Autodesk Inventor part; units mm, degrees
ref_plane "YZ Plane" through (0, 0, 0) normal (1, 0, 0) x (0, 1, 0)
ref_plane "XZ Plane" through (0, 0, 0) normal (0, 1, 0) x (-1, 0, 0)
ref_plane "XY Plane" through (0, 0, 0) normal (0, 0, 1) x (1, 0, 0)
sketch "Sketch1" plane through (0, 0, 0) normal (0, 0, 1) x (1, 0, 0)
  line L0 (0, 1490) -> (-133.543, 1490)
  line L1 (-133.543, 1490) -> (-133.543, 0)
  line L2 (-133.543, 0) -> (0, 0)
  line L3 (0, 0) -> (0, 1490)
  line L4 (-133.543, 100) -> (-66, 100)
  line L5 (-66, 100) -> (-66, 105)
  line L6 (-66, 105) -> (-133.543, 105)
  line L7 (-133.543, 105) -> (-133.543, 100)
  line L8 (-133.543, 596.6667) -> (-66, 596.6667)
  line L9 (-66, 596.6667) -> (-66, 601.6667)
  line L10 (-66, 601.6667) -> (-133.543, 601.6667)
  line L11 (-133.543, 601.6667) -> (-133.543, 596.6667)
  line L12 (-133.543, 1093.3333) -> (-66, 1093.3333)
  line L13 (-66, 1093.3333) -> (-66, 1098.3333)
  line L14 (-66, 1098.3333) -> (-133.543, 1098.3333)
  line L15 (-133.543, 1098.3333) -> (-133.543, 1093.3333)
  circle A0 centre (-133.543, 1335) radius 30
  point P0 (-133.543, 105)
  point P1 (-133.543, 1365)
  point P2 (-133.543, 1305)
  dimension "d0" = 1490
  dimension "d1" = 133.543
  dimension "d2" = 5
  dimension "d4" = 100
  dimension "d7" = 496.6667
  dimension "d23" = 66
  dimension "d29" = 60
  dimension "d30" = 1335
extrude "Plate1" add sketch "Sketch1" along normal blind 4 contours L3 L2 L1 L4 L5 L6 L8 L9 L10 L12 L13 L14 A0 L0
chamfer "Corner Chamfer1" distance 3 angle 45 6 edges at (-133.543, 100, 2) (-133.543, 105, 2) (-133.543, 596.6667, 2) (-133.543, 601.6667, 2) (-133.543, 1098.3333, 2) (-133.543, 1093.3333, 2)
equation "\"d0\" = Стрингер_длина"
equation "\"d1\" = стрингер_глубина_6"
equation "\"d2\" = паз_под_стрингер_толщина"
equation "\"d7\" = Шаг_шпангоутов"
equation "\"d23\" = паз_под_стрингер_глубина - Thickness"
equation "\"d29\" = 2 * радиус_выреза_под_сварку"
equation "\"d12\" = Thickness"
equation "\"BendRadius\" = Thickness"
equation "\"BendReliefWidth\" = Thickness"
equation "\"BendReliefDepth\" = 0.5 * Thickness"
equation "\"CornerReliefSize\" = 4 * Thickness"
equation "\"MinimumRemnant\" = 2 * Thickness"
equation "\"TransitionRadius\" = BendRadius"
equation "\"JacobiRadiusSize\" = BendRadius"
equation "\"GapSize\" = Thickness"
properties part number "0715 GBK stringer C3" material "Steel"
Could you check a few things on this model? Use its own coordinates, in mm. Give positions to 0.01 mm unless a question says otherwise; leave off trailing zeros. Order: outer loops, then holes, each group sorted by start corner. A loop starts at its lowest first (then second) coordinate and runs counter-clockwise, first axis right, second up.
Q1. Suppose I cut it at A-A, the plane y = 1335. Write out the boundary of the cut face in (x, z).
Q2. If I drill on line 1 along Y through (x, z) = (-96.5, 3.6), over which ranges is the centre line in solid material (lowest first)?
Q3. I'm going to push a flat-ended pin straight in: P1, Ø2, axis at y = 1095.5, z = 2, coming from the -X side. Where does the tip first touch, or does it pass through?
Q4. We'd pull the mould along Y, two halves only. Please class faces 1 (the cylindrical face through (-103.55, 1335.66, 1.97)), 2 (the flat face through (-68, 755, 4)): +Y half, -Y half, draft (parallel to the pull), parting line (faces both ways), or undercut.
Solution:
1. outline: (-103.54, 0) - (0, 0) - (0, 4) - (-103.54, 4) - close
2. line 1: y = 0 to 100, 105 to 596.67, 601.67 to 1093.33, 1098.33 to 1490
3. P1: stops at x = -66
4. face 1: undercut
4. face 2: draft
